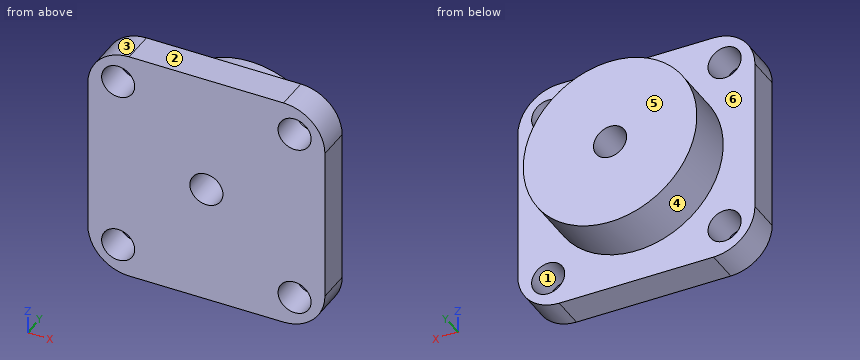
```python
from build123d import *

# Parameters (mm, degrees)
BOSS_EXTRUDE1_DEPTH = 12
SKETCH2_R           = 6
CUT_EXTRUDE1_DEPTH  = 12
SKETCH3_R           = 31.5
BOSS_EXTRUDE2_DEPTH = 18.3
SKETCH4_R           = 6
CUT_EXTRUDE2_DEPTH  = 31.3


with BuildPart() as part:
    # Sketch1 → Boss-Extrude1 (new body)
    with BuildSketch(Plane(origin=(0, 0, 0), x_dir=(1, 0, 0), z_dir=(0, 1, 0))):
        with BuildLine():
            Line((-15, 0), (-71, 0))
            ThreePointArc((-71, 0), (-81.606601718, -4.393398282), (-86, -15))
            Line((-86, -15), (-86, -71))
            ThreePointArc((-86, -71), (-81.606601718, -81.606601718), (-71, -86))
            Line((-71, -86), (-15, -86))
            ThreePointArc((-15, -86), (-4.393398282, -81.606601718), (0, -71))
            Line((0, -71), (0, -15))
            ThreePointArc((0, -15), (-4.393398282, -4.393398282), (-15, 0))
        make_face()
    extrude(amount=BOSS_EXTRUDE1_DEPTH)

    # Sketch2 → Cut-Extrude1 (cut)
    with BuildSketch(Plane(origin=(0, 12, 0), x_dir=(1, 0, 0), z_dir=(0, 1, 0))):
        with Locations((-75, -11)):
            Circle(SKETCH2_R)
        with Locations((-11, -11)):
            Circle(SKETCH2_R)
        with Locations((-11, -75)):
            Circle(SKETCH2_R)
        with Locations((-75, -75)):
            Circle(SKETCH2_R)
    extrude(amount=-CUT_EXTRUDE1_DEPTH, mode=Mode.SUBTRACT)

    # Sketch3 → Boss-Extrude2 (add)
    with BuildSketch(Plane(origin=(0, 12, 0), x_dir=(1, 0, 0), z_dir=(0, 1, 0))):
        with Locations((-43, -43)):
            Circle(SKETCH3_R)
    extrude(amount=BOSS_EXTRUDE2_DEPTH)

    # Sketch4 → Cut-Extrude2 (cut, through all)
    with BuildSketch(Plane(origin=(0, 30.3, 0), x_dir=(1, 0, 0), z_dir=(0, 1, 0))):
        with Locations((-43, -43)):
            Circle(SKETCH4_R)
    extrude(amount=-CUT_EXTRUDE2_DEPTH, mode=Mode.SUBTRACT)


solid = part.part
```
CAD build for the part. Positions are in the model's coordinates, mm. Face numbers are marked on the shaded views. A direction names the side the tool comes from. Coordinates: 2 decimals unless noted, no trailing zeros. Order: outer loops, then holes, each group sorted by start corner. A loop starts at its lowest first (then second) coordinate and runs counter-clockwise, first axis right, second up. Notation, with made-up numbers: (65.25, 3) - (69.25, 3) arc R17 cw to (69.25, 13) - close; hole circle Ø2 at (-18.5, 25). An arc over 180 degrees is marked (long way). Use a Markdown table: item, result. Add a question column.
(1) Saw through at B-B (z = 43). Give the cut face in (x, y), then the cut area to 3 significant figures.
(2) Flat gauge pins, fed straight in: pin 1 (10 mm diameter, centred on y = 11, z = 71.5, fed in from +X); pin 2 (11 mm diameter, centred on x = -11, z = 75, fed in from +Y); pin 3 (14 mm diameter, centred on x = -75, z = 75, fed in from +Y); pin 4 (8 mm diameter, centred on x = -61, y = 18.5, fed in from +Z). Where does each tip first touch, or does it go through?
(3) Pull direction X, two halves, no side cores. Call the marked faces 1, 2, 3 and 4: +X half, -X half, draft (parallel to the pull), parting line (faces both ways), or undercut.
(4) Which spindle directions (+Z, -Z, +X, -X, +Y, -Y) get a long thin tool onto all of the face, cutting with end or side? Do the marked faces 5 and 6. Say none if no direction does.
(5) Saw through at C-C (y = 6). Give the cut face in (x, z), then the cut area to 3 significant figures.
(6) Saw through at D-D (z = 19.5). Give the cut face in (x, y).
(7) Drill centre lines: line 1 along Z through (x, y) = (-42.5, 28); line 2 along Z through (x, y) = (-75, 8.5); line 3 along X through (y, z) = (3, 11). Where is each one in solid material? Low to high. Write a range as [from, to].
(8) Saw through at A-A (x = -43). Give the cut face in (y, z).
Solved:
| question | item | result |
|---|---|---|
| 1 | outline | (-86, 0) - (-49, 0) - (-49, 30.3) - (-74.5, 30.3) - (-74.5, 12) - (-86, 12) - close; (-37, 0) - (0, 0) - (0, 12) - (-11.5, 12) - (-11.5, 30.3) - (-37, 30.3) - close |
| 1 | area | 1,820 mm² |
| 2 | pin 1 | stops at x = 0 |
| 2 | pin 2 | passes through |
| 2 | pin 3 | stops at y = 12 |
| 2 | pin 4 | stops at z = 71.22 |
| 3 | face 1 | undercut |
| 3 | face 2 | draft |
| 3 | face 3 | -X half |
| 3 | face 4 | parting line |
| 4 | face 5 | +Z, -Z, +X, -X, +Y |
| 4 | face 6 | +Y |
| 5 | outline | (-86, 15) arc R15 ccw to (-71, 0) - (-15, 0) arc R15 ccw to (0, 15) - (0, 71) arc R15 ccw to (-15, 86) - (-71, 86) arc R15 ccw to (-86, 71) - close; hole circle Ø12 at (-75, 11); hole circle Ø12 at (-75, 75); hole circle Ø12 at (-43, 43); hole circle Ø12 at (-11, 11); hole circle Ø12 at (-11, 75) |
| 5 | area | 6,640 mm² |
| 6 | outline | (-86, 0) - (0, 0) - (0, 12) - (-22.02, 12) - (-22.02, 30.3) - (-63.98, 30.3) - (-63.98, 12) - (-86, 12) - close |
| 7 | line 1 | z = [11.5, 37.02], [48.98, 74.5] |
| 7 | line 2 | z = [0.54, 5], [17, 69], [81, 85.46] |
| 7 | line 3 | x = [-85.46, -81], [-69, -17], [-5, -0.54] |
| 8 | outline | (0, 0) - (12, 0) - (12, 11.5) - (30.3, 11.5) - (30.3, 37) - (0, 37) - close; (0, 49) - (30.3, 49) - (30.3, 74.5) - (12, 74.5) - (12, 86) - (0, 86) - close |
